Input: part model. Units: mm. Frame: model coordinates. A direction names the side the tool comes from. Coordinates: 2 decimals unless noted, no trailing zeros. Loops run counter-clockwise (first coordinate to the right, second up) from the corner with the lowest first, then second, coordinate; pieces in that order, holes last.
```python
from build123d import *

# Parameters (mm, degrees)
F0_R     = 18.5
F1_DEPTH = 5
F2_R     = 18.5
F2_R_2   = 15
F3_DEPTH = 14
F4_R     = 5.069848
F5_R     = 8
F5_R_2   = 3
F6_DEPTH = 14


with BuildPart() as f1:
    # F0 (on Top) → F1 (new body)
    with BuildSketch(Plane.XY):
        Circle(F0_R)
    extrude(amount=F1_DEPTH)

    # F2 (on face) → F3 (join)
    with BuildSketch(Plane.XY.offset(5)):
        Circle(F2_R)
        Circle(F2_R_2, mode=Mode.SUBTRACT)
    extrude(amount=F3_DEPTH)

    # F4
    f4_edges = [f1.edges().sort_by_distance(p)[0] for p in [
        (-18.5, 0, 0),
    ]]
    fillet(f4_edges, radius=F4_R)

    # F5 (on face) → F6 (join)
    with BuildSketch(Plane.XY.offset(5)):
        Circle(F5_R)
        Circle(F5_R_2, mode=Mode.SUBTRACT)
    extrude(amount=F6_DEPTH)


solid = f1.part
```
Item 1: Contact query for flat-ended pins moving along their axis: P1, Ø1.5, axis at y = -11, z = 2, coming from the -X side; P2, Ø3, axis at x = -0.5, y = -0.5, coming from the +Z side; P3, Ø5, axis at x = -0.5, z = 11.5, coming from the +Y side. Output: stop coordinate, or through.
Result:
P1: stops at x = -14.42
P2: stops at z = 5
P3: stops at y = 18.5
Item 2: Reachability of faces 1 (the face through (-1.73, -7.81, 11.9)), 2 (the face through (0, 0, 0)) from +Z, -Z, +X, -X, +Y, -Y: full face, straight path, thin tool, end or side. Return the list, or none.
Result:
face 1: +Z
face 2: -Z, +X, -X, +Y, -Y
Item 3: Section query A-A (x = 0). Output: boundary loops of the cut face in (y, z), then the cut area to 3 significant figures.
Result:
outline: (-18.5, 5.07) arc R5.07 ccw to (-13.43, 0) - (13.43, 0) arc R5.07 ccw to (18.5, 5.07) - (18.5, 19) - (15, 19) - (15, 5) - (8, 5) - (8, 19) - (3, 19) - (3, 5) - (-3, 5) - (-3, 19) - (-8, 19) - (-8, 5) - (-15, 5) - (-15, 19) - (-18.5, 19) - close
area: 412 mm2
Item 4: Line query: L1, parallel to Y at x = 0, z = 13.25; L2, parallel to Y at x = -6.5, z = 17; L3, parallel to Z at x = 10, y = -2. Output: solid intervals per line, ascending.
Result:
L1: y = -18.5 to -15, -8 to -3, 3 to 8, 15 to 18.5
L2: y = -17.32 to -13.52, -4.66 to 4.66, 13.52 to 17.32
L3: z = 0 to 5
Item 5: Section query B-B (z = 9.75). Output: boundary loops of the cut face in (x, y), then the cut area to 3 significant figures.
Result:
outline: circle Ø37 at (0, 0); circle Ø16 at (0, 0); hole circle Ø30 at (0, 0); hole circle Ø6 at (0, 0)
area: 541 mm2
Item 6: Mould query, pull axis X, two halves, no side actions, for faces 3 (the face through (0, 0, 5)), 4 (the face through (-0.1, 15.2, 19)), 5 (the face through (-14.985, 0.66, 11.902)), 6 (the face through (-4.01, -18.06, 11.94)). Classes: +X half, -X half, draft (parallel to the pull), parting line (faces both ways), or undercut.
Result:
face 3: undercut
face 4: draft
face 5: undercut
face 6: parting line
